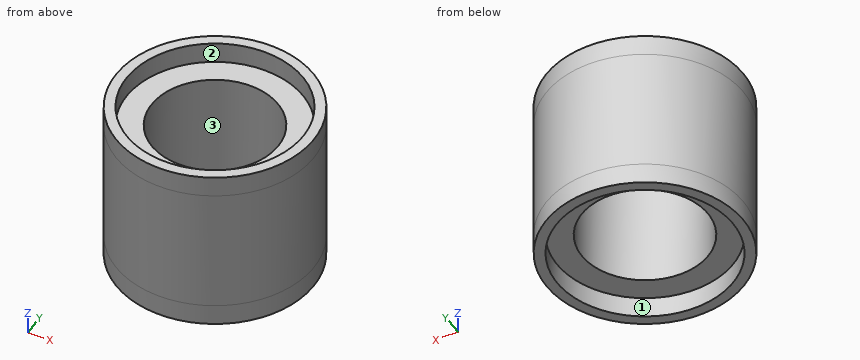
from build123d import *

# Parameters (mm, degrees)
SKETCH1_R           = 23.5
SKETCH1_R_2         = 15.05
BOSS_EXTRUDE1_DEPTH = 15
SKETCH2_R           = 23.5
SKETCH2_R_2         = 21
BOSS_EXTRUDE2_DEPTH = 5


with BuildPart() as part:
    # Sketch1 → Boss-Extrude1 (new body, symmetric)
    with BuildSketch(Plane.XY):
        Circle(SKETCH1_R)
        Circle(SKETCH1_R_2, mode=Mode.SUBTRACT)
    extrude(amount=BOSS_EXTRUDE1_DEPTH, both=True)

    # Sketch2 → Boss-Extrude2 (add)
    with BuildSketch(Plane(origin=(0, 0, -15), x_dir=(-1, 0, 0), z_dir=(0, 0, -1))):
        Circle(SKETCH2_R)
        Circle(SKETCH2_R_2, mode=Mode.SUBTRACT)
    boss_extrude2 = extrude(amount=BOSS_EXTRUDE2_DEPTH)

    # Mirror1: Boss-Extrude2 across plane
    add(boss_extrude2.mirror(Plane.XY))


solid = part.part
Geometry: final body of the model. Coordinates: model frame, mm. Face numbers are marked on the shaded views. A direction names the side the tool comes from. Coordinates: 2 decimals unless noted, no trailing zeros. Write each loop counter-clockwise with the first axis right and the second up, starting at its lowest first coordinate (ties: lowest second). Pieces come first, ordered by that corner, then holes. Notation, with made-up numbers: (76.25, -15) - (118.25, -15) arc R7 cw to (118.25, -6) - close; hole circle Ø11 at (21.25, -39). An arc over 180 degrees is marked (long way). Return JSON: item names as keys, results as strings.
Item 1: Line query: L1, parallel to Y at x = 0, z = 19; L2, parallel to Y at x = 0, z = -8.25; L3, parallel to Z at x = -19, y = 4. Output: solid intervals per line, ascending.
Completed:
{"L1": "y = -23.5 to -21, 21 to 23.5", "L2": "y = -23.5 to -15.05, 15.05 to 23.5", "L3": "z = -15 to 15"}
Item 2: Section query D-D (y = -19). Output: boundary loops of the cut face in (x, z).
Completed:
{"outline": "(-13.83, -20) - (-8.94, -20) - (-8.94, -15) - (8.94, -15) - (8.94, -20) - (13.83, -20) - (13.83, 20) - (8.94, 20) - (8.94, 15) - (-8.94, 15) - (-8.94, 20) - (-13.83, 20) - close"}
Item 3: Reachability of the marked faces 1, 2 and 3 from +Z, -Z, +X, -X, +Y, -Y: full face, straight path, thin tool, end or side. Return the list, or none.
Completed:
{"face 1": "-Z", "face 2": "+Z", "face 3": "+Z, -Z"}
Item 4: Pin query (flat end, axial travel): pin 1 Ø8 at (x, y) = (-10, -13) entering from +Z; pin 2 Ø10 at (y, z) = (-7.5, -1.5) entering from -X; pin 3 Ø25 at (x, y) = (0, 0) entering from -Z; pin 4 Ø12 at (x, z) = (15, 5.5) entering from +Y. Return the tip coordinate at first contact, or that it passes through.
Completed:
{"pin 1": "stops at z = 15", "pin 2": "stops at x = -23.37", "pin 3": "passes through", "pin 4": "stops at y = 21.71"}
Item 5: Section query C-C (z = -10). Output: boundary loops of the cut face in (x, y), and give its area (3 significant figures).
Completed:
{"outline": "circle Ø47 at (0, 0); hole circle Ø30.1 at (0, 0)", "area": "1,020 mm2"}
Item 6: Section query A-A (y = 0). Output: boundary loops of the cut face in (x, z).
Completed:
{"outline": "(-23.5, -20) - (-21, -20) - (-21, -15) - (-15.05, -15) - (-15.05, 15) - (-21, 15) - (-21, 20) - (-23.5, 20) - close; (15.05, -15) - (21, -15) - (21, -20) - (23.5, -20) - (23.5, 20) - (21, 20) - (21, 15) - (15.05, 15) - close"}
